CAD build for the part. Positions are in the model's coordinates, mm. A direction names the side the tool comes from. Coordinates: 2 decimals unless noted, no trailing zeros. Write each loop counter-clockwise with the first axis right and the second up, starting at its lowest first coordinate (ties: lowest second). Pieces come first, ordered by that corner, then holes.
```python
from build123d import *

# Parameters (mm, degrees)
PAD_DEPTH       = 44
PAD001_DEPTH    = 11.8
SKETCH002_R     = 1.7
PAD002_DEPTH    = 2
POCKET_DEPTH    = 5
SKETCH004_W     = 36
SKETCH004_H     = 34
POCKET001_DEPTH = 3
SKETCH005_W     = 36
SKETCH005_H     = 34
POCKET002_DEPTH = 4
PAD003_DEPTH    = 11.8
SKETCH007_R     = 1.7
PAD004_DEPTH    = 2
POCKET003_DEPTH = 2
PAD005_DEPTH    = 11.8
SKETCH010_R     = 1.7
PAD006_DEPTH    = 2
SKETCH011_W     = 8.8
SKETCH011_H     = 42
POCKET004_DEPTH = 2
SKETCH012_W     = 36
SKETCH012_H     = 34
POCKET005_DEPTH = 3
PAD007_DEPTH    = 15
SKETCH014_R     = 1.75
PAD008_DEPTH    = 2


with BuildPart() as part:
    # Sketch → Pad (new body)
    with BuildSketch(Plane.XY):
        Polygon((26.5581123827, 0), (-13.2790561914, 23), (-13.2790561914, -23), align=None)
        Polygon((22.5166604984, 0), (-11.2583302492, 19.5), (-11.2583302492, -19.5), align=None, mode=Mode.SUBTRACT)
    extrude(amount=PAD_DEPTH)

    # Sketch001 (on Face3 of Pad) → Pad001 (join)
    with BuildSketch(Plane(origin=(6.6395280957, -11.5, 0), x_dir=(0.8660254038, 0.5, 0), z_dir=(0.5, -0.8660254038, 0))):
        Polygon((-23, 0), (-21, 0), (-21, 42), (21, 42), (21, 0), (23, 0), (23, 44), (-23, 44), align=None)
    extrude(amount=PAD001_DEPTH)

    # Sketch002 (on Face8 of Pad001) → Pad002 (join)
    with BuildSketch(Plane(origin=(12.5395280957, -21.7190997647, 0), x_dir=(0.8660254038, 0.5, 0), z_dir=(0.5, -0.8660254038, 0))):
        Polygon((-23, 0), (-12.5, 0), (-12.5, 33.5), (12.5, 33.5), (12.5, 0), (23, 0), (23, 44), (-23, 44), align=None)
        with Locations((-15.5, 36.5)):
            Circle(SKETCH002_R, mode=Mode.SUBTRACT)
        with Locations((-15.5, 5.5)):
            Circle(SKETCH002_R, mode=Mode.SUBTRACT)
        with Locations((15.5, 5.5)):
            Circle(SKETCH002_R, mode=Mode.SUBTRACT)
        with Locations((15.5, 36.5)):
            Circle(SKETCH002_R, mode=Mode.SUBTRACT)
    extrude(amount=PAD002_DEPTH)

    # Sketch003 (on Face7 of Pad002) → Pocket (cut)
    with BuildSketch(Plane.XY.offset(44)):
        Polygon((-11.5470053838, -22), (-7.1470053838, -29.6210235533), (29.2260615752, -8.6210235533), (24.8260615752, -1), align=None)
    extrude(amount=-POCKET_DEPTH, mode=Mode.SUBTRACT)

    # Sketch004 (on Face11 of Pocket) → Pocket001 (cut)
    with BuildSketch(Plane(origin=(6.6395280957, -11.5, 0), x_dir=(0.8660254038, 0.5, 0), z_dir=(0.5, -0.8660254038, 0))):
        with Locations((0, 22)):
            Rectangle(SKETCH004_W, SKETCH004_H)
    extrude(amount=-POCKET001_DEPTH, mode=Mode.SUBTRACT)

    # Sketch005 (on Face1 of Pocket001) → Pocket002 (cut)
    with BuildSketch(Plane(origin=(6.6395280957, 11.5, 0), x_dir=(-0.8660254038, 0.5, 0), z_dir=(0.5, 0.8660254038, 0))):
        with Locations((0, 22)):
            Rectangle(SKETCH005_W, SKETCH005_H)
    extrude(amount=-POCKET002_DEPTH, mode=Mode.SUBTRACT)

    # Sketch006 (on Face1 of Pocket002) → Pad003 (join)
    with BuildSketch(Plane(origin=(6.6395280957, 11.5, 0), x_dir=(-0.8660254038, 0.5, 0), z_dir=(0.5, 0.8660254038, 0))):
        Polygon((-23, 44), (23, 44), (23, 0), (21, 0), (21, 42), (-21, 42), (-21, 0), (-23, 0), align=None)
    extrude(amount=PAD003_DEPTH)

    # Sketch007 (on Face19 of Pad003) → Pad004 (join)
    with BuildSketch(Plane(origin=(12.5395280957, 21.7190997647, 0), x_dir=(-0.8660254038, 0.5, 0), z_dir=(0.5, 0.8660254038, 0))):
        Polygon((-23, 0), (-12.5, 0), (-12.5, 33.5), (12.5, 33.5), (12.5, 0), (23, 0), (23, 44), (-23, 44), align=None)
        with Locations((-15.5, 36.5)):
            Circle(SKETCH007_R, mode=Mode.SUBTRACT)
        with Locations((15.5, 36.5)):
            Circle(SKETCH007_R, mode=Mode.SUBTRACT)
        with Locations((15.5, 5.5)):
            Circle(SKETCH007_R, mode=Mode.SUBTRACT)
        with Locations((-15.5, 5.5)):
            Circle(SKETCH007_R, mode=Mode.SUBTRACT)
    extrude(amount=PAD004_DEPTH)

    # Sketch008 (on Face43 of Pad004) → Pocket003 (cut)
    with BuildSketch(Plane.XY.offset(44)):
        Polygon((-11.5470053838, 22), (-7.1470053838, 29.6210235533), (29.2260615751, 8.6210235533), (24.8260615752, 1), align=None)
    extrude(amount=-POCKET003_DEPTH, mode=Mode.SUBTRACT)

    # Sketch009 (on Face12 of Pocket003) → Pad005 (join)
    with BuildSketch(Plane(origin=(-13.2790561914, 0, 0), x_dir=(0, -1, 0), z_dir=(-1, 0, 0))):
        Polygon((-23, 0), (-21, 0), (-21, 42), (21, 42), (21, 0), (23, 0), (23, 44), (-23, 44), align=None)
    extrude(amount=PAD005_DEPTH)

    # Sketch010 (on Face32 of Pad005) → Pad006 (join)
    with BuildSketch(Plane(origin=(-25.0790561914, 0, 0), x_dir=(0, -1, 0), z_dir=(-1, 0, 0))):
        Polygon((-23, 0), (-12.5, 0), (-12.5, 33.5), (12.5, 33.5), (12.5, 0), (23, 0), (23, 44), (-23, 44), align=None)
        with Locations((-15.5, 5.5)):
            Circle(SKETCH010_R, mode=Mode.SUBTRACT)
        with Locations((-15.5, 36.5)):
            Circle(SKETCH010_R, mode=Mode.SUBTRACT)
        with Locations((15.5, 36.5)):
            Circle(SKETCH010_R, mode=Mode.SUBTRACT)
        with Locations((15.5, 5.5)):
            Circle(SKETCH010_R, mode=Mode.SUBTRACT)
    extrude(amount=PAD006_DEPTH)

    # Sketch011 (on Face57 of Pad006) → Pocket004 (cut)
    with BuildSketch(Plane.XY.offset(44)):
        with Locations((-17.6790561914, 0)):
            Rectangle(SKETCH011_W, SKETCH011_H)
    extrude(amount=-POCKET004_DEPTH, mode=Mode.SUBTRACT)

    # Sketch012 (on Face13 of Pocket004) → Pocket005 (cut)
    with BuildSketch(Plane(origin=(-13.2790561914, 0, 0), x_dir=(0, -1, 0), z_dir=(-1, 0, 0))):
        with Locations((0, 22)):
            Rectangle(SKETCH012_W, SKETCH012_H)
    extrude(amount=-POCKET005_DEPTH, mode=Mode.SUBTRACT)

    # Sketch013 (on Face25 of Pocket005) → Pad007 (join)
    with BuildSketch(Plane.XY.offset(44)):
        Polygon((-13.2790561914, 21), (-11.5470053838, 22), (24.8260615752, 1), (24.8260615752, -1), (-11.5470053838, -22), (-13.2790561914, -21), align=None)
        Polygon((-11.2583302492, 19.5), (22.5166604984, 0), (-11.2583302492, -19.5), align=None, mode=Mode.SUBTRACT)
    extrude(amount=PAD007_DEPTH)

    # Sketch014 (on Face66 of Pad007) → Pad008 (join)
    with BuildSketch(Plane.XY.offset(59)):
        Polygon((-13.2790561914, 21), (-11.5470053838, 22), (24.8260615752, 1), (24.8260615752, -1), (-11.5470053838, -22), (-13.2790561914, -21), align=None)
        with Locations((-7.2790561914, 0)):
            Circle(SKETCH014_R, mode=Mode.SUBTRACT)
        with Locations((3.6395280957, 6.3038475773)):
            Circle(SKETCH014_R, mode=Mode.SUBTRACT)
        with Locations((3.6395280957, -6.3038475773)):
            Circle(SKETCH014_R, mode=Mode.SUBTRACT)
        Polygon((6.5581123827, 0), (-3.2790561914, 5.6794919243), (-3.2790561914, -5.6794919243), align=None, mode=Mode.SUBTRACT)
    extrude(amount=PAD008_DEPTH)


solid = part.part
```
Item 1: Wall check: line 1 along Z through (x, y) = (-26, -15.5); line 2 along Y through (x, z) = (-23, 40); line 3 along Y through (x, z) = (18, 42.5). Give the ranges that are in metal, low to high.
Item 2: Two-plate mould, pull along Z, no slides. Class faces 5 (the flat face through (15, -18, 44)), 6 (the cylindrical face through (-0.71, -30.51, 34.84)), 7 (the cylindrical face through (3.41, 8.04, 59.99)): +Z half, -Z half, draft (parallel to the pull), parting line (faces both ways), or undercut.
Item 3: Saw through at B-B, the plane x = 19.5. Write the cut outline in (y, z) (3 decimals), and give its area (3 significant figures).
Item 4: Flat gauge pins, fed straight in: pin 1 Ø1.6 at (x, z) = (-12.5, 24.5) entering from -Y (3 decimals); pin 2 Ø2 at (x, y) = (8.5, -23.5) entering from +Z; pin 3 Ø5 at (x, z) = (-11, 7) entering from -Y; pin 4 Ø3 at (x, y) = (-7.28, 0) entering from +Z. Where does each tip first touch, or does it go through?
Item 5: Saw through at A-A, the plane x = -19.5. Write the cut outline in (y, z).
Item 6: Which spindle directions (+Z, -Z, +X, -X, +Y, -Y) get a long thin tool onto all of the face, cutting with end or side? Do faces 1 (the flat face through (23.858, 16.323, 16.516)), 2 (the flat face through (6, -11, 39)), 3 (the flat face through (2, 5, 59)), 4 (the flat face through (-20, -23, 22)). Say none if no direction does.
Working result:
1. line 1: z = 0 to 3.8, 7.2 to 34.8, 38.2 to 44
1. line 2: y = -23 to -21, 21 to 23
1. line 3: y = -20.88 to -15.1, -4.94 to -2.61, 2.61 to 4.94, 15.1 to 20.88
2. face 5: +Z half
2. face 6: undercut
2. face 7: draft
3. outline: (-20.01, 33.5) - (-17.7, 33.5) - (-17.7, 42) - (-14.236, 42) - (-14.236, 44) - (-20.01, 44) - close; (-4.075, 0) - (-1.742, 0) - (-1.742, 5) - (-4.075, 5) - close; (-4.075, 39) - (-1.742, 39) - (-1.742, 59) - (1.742, 59) - (1.742, 39) - (4.075, 39) - (4.075, 61) - (-4.075, 61) - close; (1.742, 0) - (4.075, 0) - (4.075, 5) - (1.742, 5) - close; (14.236, 42) - (17.7, 42) - (17.7, 33.5) - (20.01, 33.5) - (20.01, 44) - (14.236, 44) - close
3. area: 195 mm2
4. pin 1: stops at y = -25.735
4. pin 2: stops at z = 44
4. pin 3: stops at y = -31.28
4. pin 4: passes through
5. outline: (-23, 0) - (-21, 0) - (-21, 44) - (-23, 44) - close; (21, 0) - (23, 0) - (23, 44) - (21, 44) - close
6. face 1: -Z, +Y
6. face 2: none
6. face 3: -Z
6. face 4: +Z, -Z, -X, -Y
